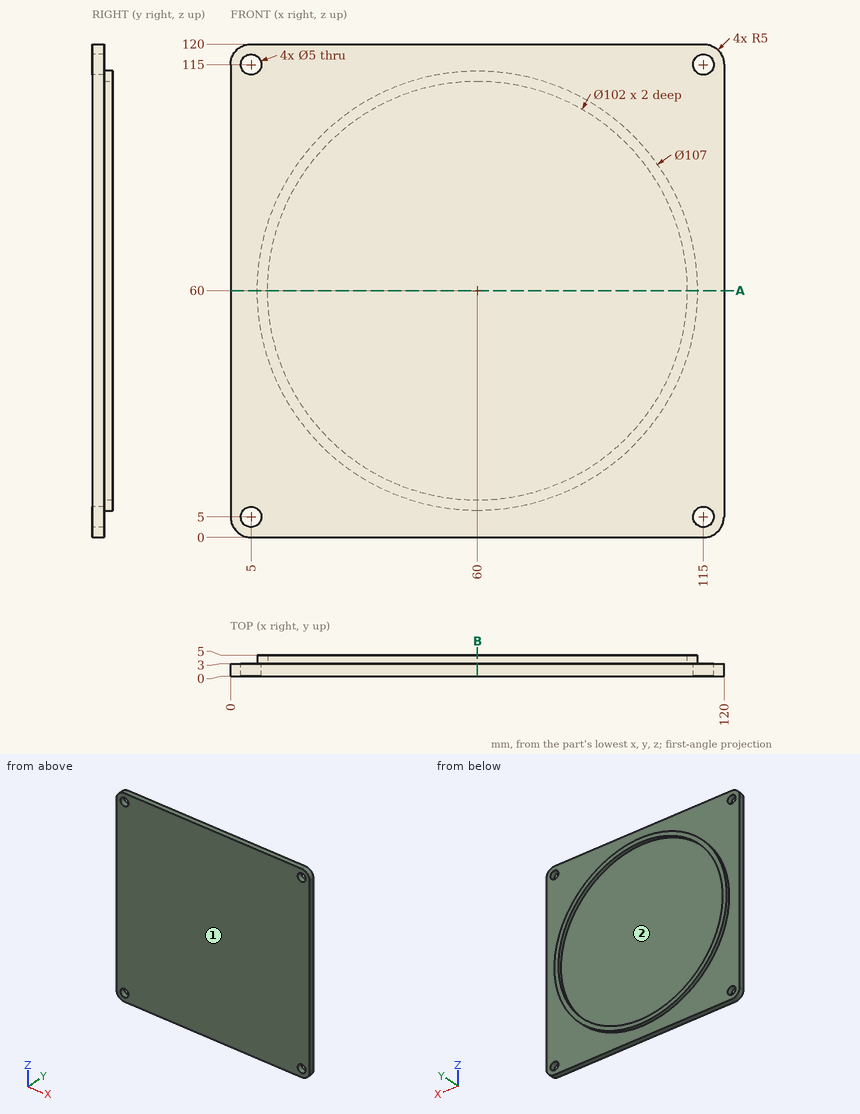
Could you check a few things on this drawing? It's one solid part, dimensions in mm from its lowest x, y, z. Coordinates: 2 decimals unless noted, no trailing zeros. Order: outer loops, then holes, each group sorted by start corner. A loop starts at its lowest first (then second) coordinate and runs counter-clockwise, first axis right, second up. Notation, with made-up numbers: M 57.5,-26 L 70.5,-26 A12 cw 70.5,-10 Z; hole C 17,34 d8. An arc over 180 degrees is marked long. Use a Markdown table: item, result. Add a question column.
Q1. We'd pull the mould along X, two halves only. Please class the marked faces 1 and 2: pulls with the +X half, pulls with the -X half, needs draft (parallel to the pull), parting line crosses it, or undercut.
Q2. If I drill on L1, parallel to X at y = 1.15, z = 5; L2, parallel to Y at x = 95.5, z = 40; L3, parallel to Z at x = 114.5, y = 1.35, over which ranges is the centre line in solid material (lowest first)?
Q3. I'm going to push flat-ended pins straight in: pin 1 (1.5 mm diameter, centred on x = 14, y = 4, fed in from -Z); pin 2 (6.5 mm diameter, centred on x = 5, z = 115, fed in from +Y). Where does each tip first touch, or does it pass through?
Q4. I want a section at B-B on x = 60. List the corners of the cut face in (y, z) for me, then the cut area to 3 significant figures.
Q5. I want a section at A-A on z = 60. List the corners of the cut face in (x, y) for me.
Checked values:
| question | item | result |
|---|---|---|
| 1 | face 1 | needs draft |
| 1 | face 2 | undercut |
| 2 | L1 | 0 to 2.5, 7.5 to 112.5, 117.5 to 120 |
| 2 | L2 | 0 to 3 |
| 2 | L3 | 0 to 2.55, 7.45 to 112.55, 117.45 to 120 |
| 3 | pin 1 | z = 31.46 |
| 3 | pin 2 | y = 3 |
| 4 | outline | M 0,0 L 3,0 L 3,6.5 L 5,6.5 L 5,9 L 3,9 L 3,111 L 5,111 L 5,113.5 L 3,113.5 L 3,120 L 0,120 Z |
| 4 | area | 370 mm² |
| 5 | outline | M 0,0 L 120,0 L 120,3 L 113.5,3 L 113.5,5 L 111,5 L 111,3 L 9,3 L 9,5 L 6.5,5 L 6.5,3 L 0,3 Z |
